Part print with two shaded views. Sizes in mm from the minimum x, y, z corner. A direction names the side the tool comes from. Round coordinates to 2 decimals unless told otherwise and drop trailing zeros. Loops run counter-clockwise (first coordinate to the right, second up) from the corner with the lowest first, then second, coordinate; pieces in that order, holes last. Notation, with made-up numbers: (33.25, 28) - (63.25, 28) arc R31 cw to (63.25, 55) - close; hole circle Ø4 at (-29, 39.25). An arc over 180 degrees is marked (long way). Use a Markdown table: item, result.
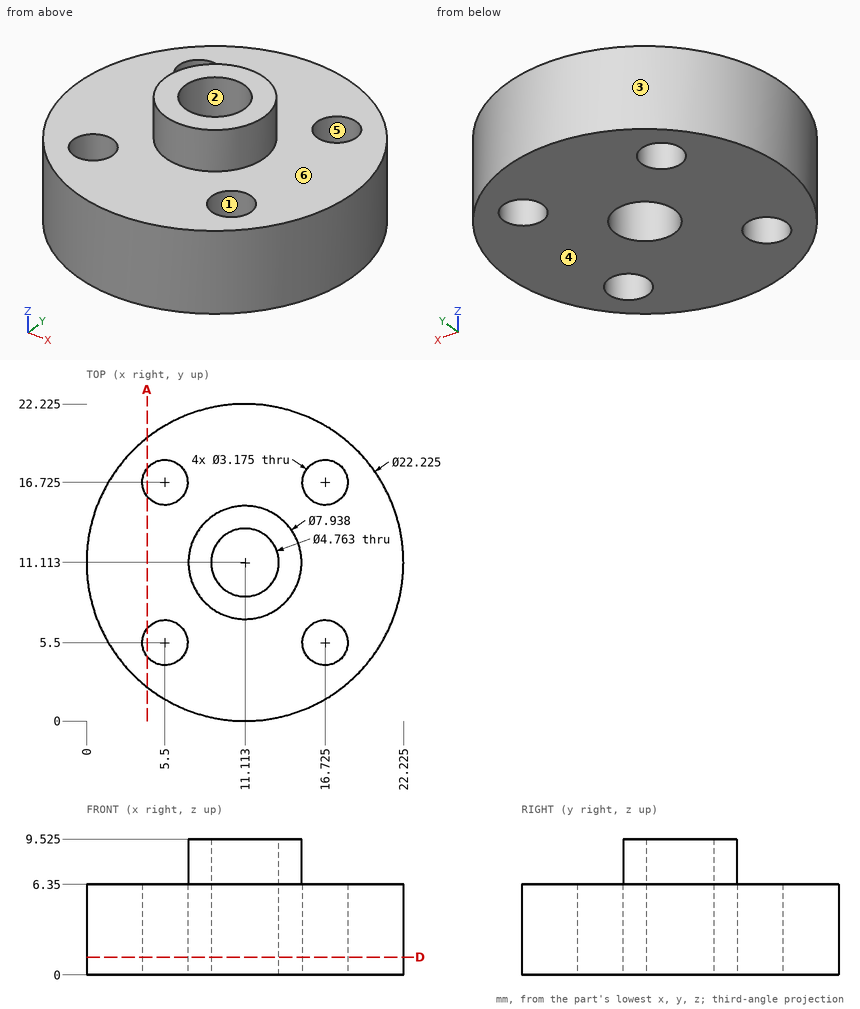
Q1. Cut at A-A, the plane x = 4.25. List the corners of the cut face in (y, z).
Results found:
| item | result |
|---|---|
| outline | (2.37, 0) - (4.52, 0) - (4.52, 6.35) - (2.37, 6.35) - close; (6.48, 0) - (15.75, 0) - (15.75, 6.35) - (6.48, 6.35) - close; (17.7, 0) - (19.85, 0) - (19.85, 6.35) - (17.7, 6.35) - close |
Q2. Pull direction X, two halves, no side cores. Call the marked faces 1, 2, 3 and 4: pulls with the +X half, pulls with the -X half, needs draft (parallel to the pull), parting line crosses it, or undercut.
Results found:
| item | result |
|---|---|
| face 1 | undercut |
| face 2 | undercut |
| face 3 | parting line crosses it |
| face 4 | needs draft |
Q3. Drop flat-ended pins along their axis: pin 1 (8 mm diameter, centred on x = 16.5, y = 5.5, fed in from +Z) (1 decimal); pin 2 (3 mm diameter, centred on x = 13, z = 1.5, fed in from -Y); pin 3 (1.5 mm diameter, centred on y = 8.5, z = 3, fed in from -X); pin 4 (4 mm diameter, centred on y = 9, z = 7, fed in from +X). Give the stop position or say it passes through.
Results found:
| item | result |
|---|---|
| pin 1 | stops at z = 9.5 |
| pin 2 | stops at y = 0.01 |
| pin 3 | stops at x = 0.16 |
| pin 4 | stops at x = 22.22 |
Q4. Which spindle directions (+Z, -Z, +X, -X, +Y, -Y) get a long thin tool onto all of the face, cutting with end or side? Do the marked faces 5 and 6. Say none if no direction does.
Results found:
| item | result |
|---|---|
| face 5 | +Z, -Z |
| face 6 | +Z |
Q5. Probe line 1 (X direction, y = 11.25, z = 8.25) (1 decimal); line 2 (Y direction, x = 6.5, z = 2) (1 decimal); line 3 (X direction, y = 17.5, z = 5) (1 decimal). List the from-to ranges inside material, lowest first.
Results found:
| item | result |
|---|---|
| line 1 | x = 7.1 to 8.7, 13.5 to 15.1 |
| line 2 | y = 1 to 4.3, 6.7 to 15.5, 18 to 21.2 |
| line 3 | x = 2 to 4.1, 6.9 to 15.3, 18.1 to 20.2 |
Q6. Cut at D-D, the plane z = 1.25. List the corners of the cut face in (x, y) (1 decimal).
Results found:
| item | result |
|---|---|
| outline | circle Ø22.2 at (11.1, 11.1); hole circle Ø3.2 at (5.5, 5.5); hole circle Ø3.2 at (5.5, 16.7); hole circle Ø4.8 at (11.1, 11.1); hole circle Ø3.2 at (16.7, 5.5); hole circle Ø3.2 at (16.7, 16.7) |
